Build history of the part. All positions in model axes, mm. A direction names the side the tool comes from. Round coordinates to 2 decimals unless told otherwise and drop trailing zeros. Order: outer loops, then holes, each group sorted by start corner. A loop starts at its lowest first (then second) coordinate and runs counter-clockwise, first axis right, second up. Notation, with made-up numbers: (70.5, -38) -> (125.5, -38) arc R37 cw to (125.5, -2) -> close; hole circle Ø3 at (-20, -4). An arc over 180 degrees is marked (long way). Answer as CSV lines item,"result". Start each with the question number.
```python
from build123d import *

# Parameters (mm, degrees)
F1_DEPTH = 10
F2_R     = 10
F3_DEPTH = 20
F5_DEPTH = 5


with BuildPart() as f1:
    # F0 (on Top) → F1 (new body)
    with BuildSketch(Plane.XY):
        with BuildLine():
            Line((51.441539079, 20), (0, 20))
            ThreePointArc((0, 20), (-20, 0), (0, -20))
            ThreePointArc((0, -20), (0.030776405, -19.9999763203), (0.061552737, -19.9999052813))
            Line((0.061552737, -19.9999052813), (49.6942619614, -19.9235293729))
            Line((49.6942619614, -19.9235293729), (53.2501253097, -19.9180575319))
            ThreePointArc((53.2501253097, -19.9180575319), (71.4210429597, 0.905220791), (51.441539079, 20))
        make_face()
    extrude(amount=F1_DEPTH)

    # F2 (on face) → F3 (join)
    with BuildSketch(Plane.XY.offset(10)):
        with BuildLine():
            ThreePointArc((0.061552737, -19.9999052813), (14.1638810843, -14.120356675), (20, 0))
            ThreePointArc((20, 0), (14.1421356237, 14.1421356237), (0, 20))
            ThreePointArc((0, 20), (-20, 0), (0, -20))
            ThreePointArc((0, -20), (0.030776405, -19.9999763203), (0.061552737, -19.9999052813))
        make_face()
        Circle(F2_R, mode=Mode.SUBTRACT)
    extrude(amount=F3_DEPTH)

    # F4 (on face) → F5 (cut)
    with BuildSketch(Plane.XY.offset(30)):
        with BuildLine():
            Line((-6.6143782777, 7.5), (-18.5404962177, 7.5))
            ThreePointArc((-18.5404962177, 7.5), (-20, 0), (-18.5404962177, -7.5))
            Line((-18.5404962177, -7.5), (-6.6143782777, -7.5))
            ThreePointArc((-6.6143782777, -7.5), (-10, 0), (-6.6143782777, 7.5))
        make_face()
        with BuildLine():
            ThreePointArc((20, 0), (19.63173355, 3.8203452491), (18.5404962177, 7.5))
            Line((18.5404962177, 7.5), (6.6143782777, 7.5))
            ThreePointArc((6.6143782777, 7.5), (9.1143782777, 4.1143782777), (10, 0))
            ThreePointArc((10, 0), (9.1143782777, -4.1143782777), (6.6143782777, -7.5))
            Line((6.6143782777, -7.5), (18.5404962177, -7.5))
            ThreePointArc((18.5404962177, -7.5), (19.63173355, -3.8203452491), (20, 0))
        make_face()
    extrude(amount=-F5_DEPTH, mode=Mode.SUBTRACT)


solid = f1.part
```
Q1. Slice it at C-C, the plane x = -3.5. Write the cut outline in (y, z), plus the area to 3 significant figures.
Q2. Which spindle directions (+Z, -Z, +X, -X, +Y, -Y) get a long thin tool onto all of the face, cutting with end or side? Do faces 4 (the face through (0, 14, 30)), 5 (the face through (9.54, 3, 19.86)), 6 (the face through (15, 0, 25)). Say none if no direction does.
Q3. Flat gauge pins, fed straight in: pin 1 Ø10 at (x, y) = (-9.5, 5.5) entering from +Z; pin 2 Ø4 at (x, z) = (12, 26.5) entering from -Y; pin 3 Ø20 at (x, y) = (34.5, 5.5) entering from +Z; pin 4 Ø2.5 at (x, z) = (12, 28.5) entering from +Y. Where does each tip first touch, or does it go through?
Q4. Two-plate mould, pull along X, no slides. Class faces 1 (the face through (26, 20, 5)), 2 (the face through (71.436, 0.478, 4.93)), 3 (the face through (0, 0, 10)): +X half, -X half, draft (parallel to the pull), parting line (faces both ways), or undercut.
Q5. Slice it at D-D, the plane y = 17. Write the cut outline in (x, z).
Q6. Slice it at B-B, the plane z = 7. Write the cut outline in (x, y).
Q7. Slice it at A-A, the plane z = 26. Write the cut outline in (x, y).
Q8. Probe L1, parallel to Z at x = 46, y = -13; L2, parallel to X at y = -4.5, z = 21; L3, parallel to Y at x = 50, z = 8.5. List the from-to ranges inside material, lowest first.
Solutions:
1,outline,"(-19.69, 0) -> (19.69, 0) -> (19.69, 30) -> (9.37, 30) -> (9.37, 10) -> (-9.37, 10) -> (-9.37, 30) -> (-19.69, 30) -> close"
1,area,"807 mm2"
2,face 4,"+Z, +X, -X, +Y, -Y"
2,face 5,"+Z"
2,face 6,"+Z, +X, -X"
3,pin 1,"stops at z = 30"
3,pin 2,"stops at y = -17.32"
3,pin 3,"stops at z = 10"
3,pin 4,"stops at y = 16.87"
4,face 1,"draft"
4,face 2,"+X half"
4,face 3,"undercut"
5,outline,"(-10.54, 0) -> (61.98, 0) -> (61.98, 10) -> (10.54, 10) -> (10.54, 30) -> (-10.54, 30) -> close"
6,outline,"(0, -20) arc R20 ccw to (0.06, -20) -> (53.25, -19.92) arc R20 ccw to (51.44, 20) -> (0, 20) arc R20 ccw to start"
7,outline,"(-18.54, -7.5) arc R20 ccw to (0, -20) arc R20 ccw to (0.06, -20) arc R20 ccw to (18.54, -7.5) -> (6.61, -7.5) arc R10 cw to (-6.61, -7.5) -> close; (-18.54, 7.5) -> (-6.61, 7.5) arc R10 cw to (6.61, 7.5) -> (18.54, 7.5) arc R20 ccw to start"
8,L1,"z = 0 to 10"
8,L2,"x = -19.49 to -8.93, 8.93 to 19.49"
8,L3,"y = -19.92 to 20"
